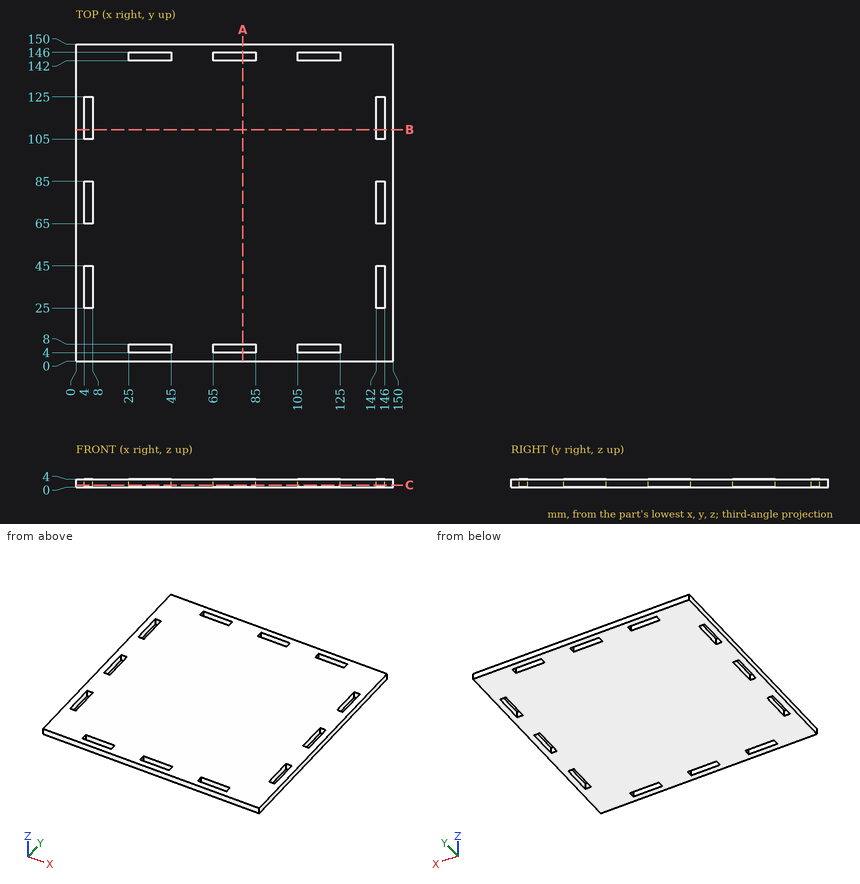
Design review of the part shown in the three views and the two pictorial views. Dimensions are in mm from the part's minimum x, y and z. Coordinates: 2 decimals unless noted, no trailing zeros. Loops run counter-clockwise (first coordinate to the right, second up) from the corner with the lowest first, then second, coordinate; pieces in that order, holes last. Notation, with made-up numbers: (-20.75, 54.25) - (7.25, 54.25) arc R15 cw to (7.25, 69.25) - close; hole circle Ø2 at (-30.5, 74). An arc over 180 degrees is marked (long way). Use a Markdown table: item, result. Add a question column.
Item 1: We need section A-A (x = 79). Give the boundary of the cut face in (y, z), and give its area (3 significant figures).
Item 2: We need section C-C (z = 1.1). Give the number of separate pieces and of enclosed holes in the cut face, and give its area (3 significant figures).
Item 3: For line 1 (Y direction, x = 123.5, z = 0.45); line 2 (X direction, y = 143, z = 2.1), list the stretches that pass through material, from the lowest coordinate up.
Results list:
| question | item | result |
|---|---|---|
| 1 | outline | (0, 0) - (4, 0) - (4, 4) - (0, 4) - close; (8, 0) - (142, 0) - (142, 4) - (8, 4) - close; (146, 0) - (150, 0) - (150, 4) - (146, 4) - close |
| 1 | area | 568 mm^2 |
| 2 | separate pieces | 1 |
| 2 | enclosed holes | 12 |
| 2 | area | 21,500 mm^2 |
| 3 | line 1 | y = 0 to 4, 8 to 142, 146 to 150 |
| 3 | line 2 | x = 0 to 25, 45 to 65, 85 to 105, 125 to 150 |
